The drawing under review shows one solid part. Ordinate dimensions are in mm from its lowest x, y, z. A direction names the side the tool comes from. Coordinates: 2 decimals unless noted, no trailing zeros. Loops run counter-clockwise (first coordinate to the right, second up) from the corner with the lowest first, then second, coordinate; pieces in that order, holes last. Notation, with made-up numbers: M -23.75,-30 L 30.25,-30 A9 ccw 30.25,-19 Z; hole C 43.5,40 d1. An arc over 180 degrees is marked long. Return JSON: item names as keys, results as strings.
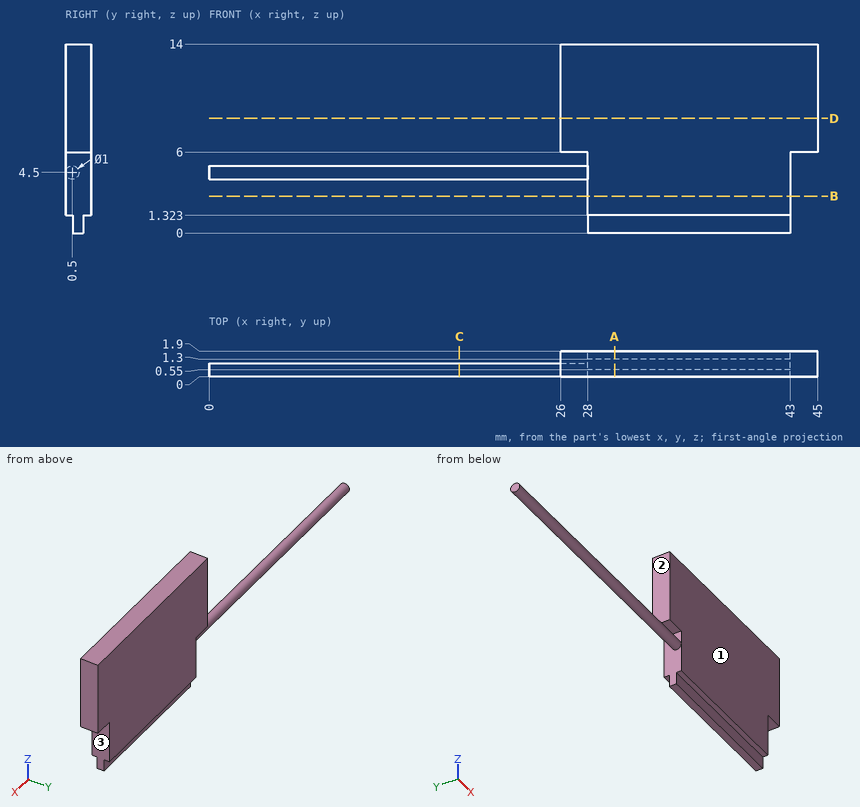
1. To check wall thickness, follow line 1 (X direction, y = 0.15, z = 5.25); line 2 (X direction, y = 1.1, z = 12.75); line 3 (Y direction, x = 37, z = 1.25). State the ranges of each line that lie inside material, in increasing order.
Check values:
{"line 1": "28 to 43", "line 2": "26 to 45", "line 3": "0.55 to 1.3"}
2. Insertion check: pin 1 Ø5 at (x, z) = (7, 4.5) entering from +Y; pin 2 Ø0.6 at (x, y) = (38.5, 0.5) entering from -Z; pin 3 Ø0.6 at (y, z) = (1, 10.5) entering from -X; pin 4 Ø0.6 at (y, z) = (1.5, 2.5) entering from +X. Each pin has a flat end and moves straight along its axis. Give the tip position at first contact, or say it passes through.
Check values:
{"pin 1": "y = 1", "pin 2": "z = 0", "pin 3": "x = 26", "pin 4": "x = 43"}
3. Add section A-A on x = 30. Give the boundary of the cut face in (y, z).
Check values:
{"outline": "M 0,1.32 L 0.55,1.32 L 0.55,0 L 1.3,0 L 1.3,1.32 L 1.9,1.32 L 1.9,14 L 0,14 Z"}
4. Add section C-C on x = 18.5. Give the boundary of the cut face in (y, z).
Check values:
{"outline": "C 0.5,4.5 d1"}
5. Add section D-D on z = 8.5. Give the boundary of the cut face in (x, y), plus the area to 3 significant figures.
Check values:
{"outline": "M 26,0 L 45,0 L 45,1.9 L 26,1.9 Z", "area": "36.1 mm²"}
6. Add section B-B on z = 2.75. Give the boundary of the cut face in (x, y), plus the area to 3 significant figures.
Check values:
{"outline": "M 28,0 L 43,0 L 43,1.9 L 28,1.9 Z", "area": "28.5 mm²"}
7. Machinability: for the marked faces 1, 2 and 3, which of the approach directions +Z, -Z, +X, -X, +Y, -Y give a long, thin tool a straight path to every point of the face, cutting with its end or side? Answer none if there is none.
Check values:
{"face 1": "+Z, -Z, +X, -X, -Y", "face 2": "+Z, -X, +Y, -Y", "face 3": "-Z, +X, +Y, -Y"}
